Part model, mm, in its own coordinate system. Give positions to 0.01 mm unless a question says otherwise; leave off trailing zeros. Write each loop counter-clockwise with the first axis right and the second up, starting at its lowest first coordinate (ties: lowest second). Pieces come first, ordered by that corner, then holes. Notation, with made-up numbers: M -21,67.5 L 8,67.5 A25 ccw 8,88.5 Z; hole C -1,-35.75 d2. An arc over 180 degrees is marked long. Use a Markdown table: item, result.
```python
from build123d import *

# Parameters (mm, degrees)
F0_R     = 3.6195
F0_R_2   = 41.94175
F1_DEPTH = 12.7
F2_W     = 71.12
F2_H     = 12.7
F3_DEPTH = 12.7
F4_R     = 3.175


with BuildPart() as f1:
    # F0 (on Top) → F1 (new body)
    with BuildSketch(Plane.XY):
        with BuildLine():
            Line((37.5943482574, 0), (-37.5943482574, 0))
            ThreePointArc((-37.5943482574, 0), (-40.5487339943, -0.3484169064), (-43.3410161187, -1.3745504066))
            Line((-43.3410161187, -1.3745504066), (-170.8466678613, -66.0724350219))
            ThreePointArc((-170.8466678614, -66.0724350219), (-175.9229543527, -70.7530626401), (-177.8, -77.3978846153))
            Line((-177.8, -77.3978846153), (-177.8, -180.8720758428))
            Line((-177.8, -180.8720758428), (177.8, -180.8720758428))
            Line((177.8, -180.8720758428), (177.8, -77.3978846153))
            ThreePointArc((177.8, -77.3978846153), (175.9229543526, -70.7530626402), (170.8466678613, -66.0724350219))
            Line((170.8466678613, -66.0724350219), (43.3410161187, -1.3745504066))
            ThreePointArc((43.3410161187, -1.3745504066), (40.5487339943, -0.3484169064), (37.5943482574, 0))
        make_face()
        with Locations((-45.3171624807, -155.4720758428)):
            Circle(F0_R, mode=Mode.SUBTRACT)
        with Locations((45.3171624807, -155.4720758428)):
            Circle(F0_R, mode=Mode.SUBTRACT)
        with Locations((-165.1, -77.3978846153)):
            Circle(F0_R, mode=Mode.SUBTRACT)
        with Locations((-82.6705035794, -81.856653486)):
            Circle(F0_R_2, mode=Mode.SUBTRACT)
        with Locations((-37.5943482574, -12.7)):
            Circle(F0_R, mode=Mode.SUBTRACT)
        with Locations((82.6705035794, -81.856653486)):
            Circle(F0_R_2, mode=Mode.SUBTRACT)
        with Locations((165.1, -77.3978846153)):
            Circle(F0_R, mode=Mode.SUBTRACT)
        with Locations((37.5943482574, -12.7)):
            Circle(F0_R, mode=Mode.SUBTRACT)
    extrude(amount=F1_DEPTH)

    # F2 (on face) → F3 (cut, through all)
    with BuildSketch(Plane.XY.offset(12.7)):
        with Locations((-142.24, -174.5220758428)):
            Rectangle(F2_W, F2_H)
        with Locations((142.24, -174.5220758428)):
            Rectangle(F2_W, F2_H)
        with Locations((0, -174.5220758428)):
            Rectangle(F2_W, F2_H)
    extrude(amount=-F3_DEPTH, mode=Mode.SUBTRACT)

    # F4
    f4_edges = [f1.edges().sort_by_distance(p)[0] for p in [
        (-177.8, -168.172076, 6.35),
        (-106.68, -168.172076, 6.35),
        (-35.56, -168.172076, 6.35),
        (35.56, -168.172076, 6.35),
        (106.68, -168.172076, 6.35),
        (177.8, -168.172076, 6.35),
        (-106.68, -180.872076, 6.35),
        (-35.56, -180.872076, 6.35),
        (35.56, -180.872076, 6.35),
        (106.68, -180.872076, 6.35),
    ]]
    fillet(f4_edges, radius=F4_R)


solid = f1.part
```
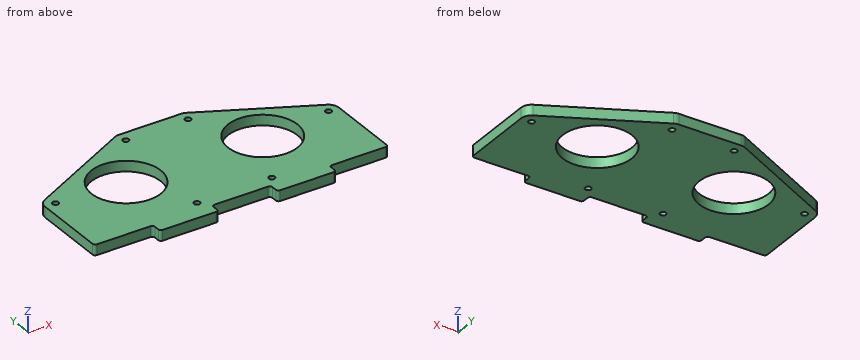
1. Cut at A-A, the plane y = -12.7. Give the cut face in (x, z), then the cut area to 3 significant figures.
Findings below:
| item | result |
|---|---|
| outline | M -65.66,0 L -41.21,0 L -41.21,12.7 L -65.66,12.7 Z; M -33.97,0 L 33.97,0 L 33.97,12.7 L -33.97,12.7 Z; M 41.21,0 L 65.66,0 L 65.66,12.7 L 41.21,12.7 Z |
| area | 1,480 mm2 |
2. Drill centre lines: L1, parallel to X at y = -61, z = 3.25; L2, parallel to X at y = -47, z = 10.5; L3, parallel to Y at x = -165.1, z = 4. Where is each one in solid material? Low to high.
Findings below:
| item | result |
|---|---|
| L1 | -160.85 to -119.06, -46.28 to 46.28, 119.06 to 160.85 |
| L2 | -133.26 to -106, -59.34 to 59.34, 106 to 133.26 |
| L3 | -168.17 to -81.02, -73.78 to -63.16 |
3. Cut at D-D, the plane z = 5. State how many separate pieces and enclosed holes the cut face has, then the cut area to 3 significant figures.
Findings below:
| item | result |
|---|---|
| separate pieces | 1 |
| enclosed holes | 8 |
| area | 40,700 mm2 |
4. Cut at B-B, the plane x = 165.1. Give the cut face in (y, z).
Findings below:
| item | result |
|---|---|
| outline | M -168.17,0 L -81.02,0 L -81.02,12.7 L -168.17,12.7 Z; M -73.78,0 L -63.16,0 L -63.16,12.7 L -73.78,12.7 Z |
5. Drop flat-ended pins along their axis: P1, Ø6.5, axis at x = 142, z = 8.5, coming from the -Y side; P2, Ø8.5, axis at x = 45.32, y = -155.47, coming from the +Z side; P3, Ø5, axis at x = -107, z = 9, coming from the -Y side; P4, Ø5, axis at y = -176, z = 4, coming from the -X side. Give the stop position or say it passes through.
Findings below:
| item | result |
|---|---|
| P1 | y = -168.17 |
| P2 | z = 12.7 |
| P3 | y = -180.71 |
| P4 | x = -106.68 |
6. Cut at C-C, the plane y = -55. Give the cut face in (x, z).
Findings below:
| item | result |
|---|---|
| outline | M -149.03,0 L -114.89,0 L -114.89,12.7 L -149.03,12.7 Z; M -50.46,0 L 50.46,0 L 50.46,12.7 L -50.46,12.7 Z; M 114.89,0 L 149.03,0 L 149.03,12.7 L 114.89,12.7 Z |
